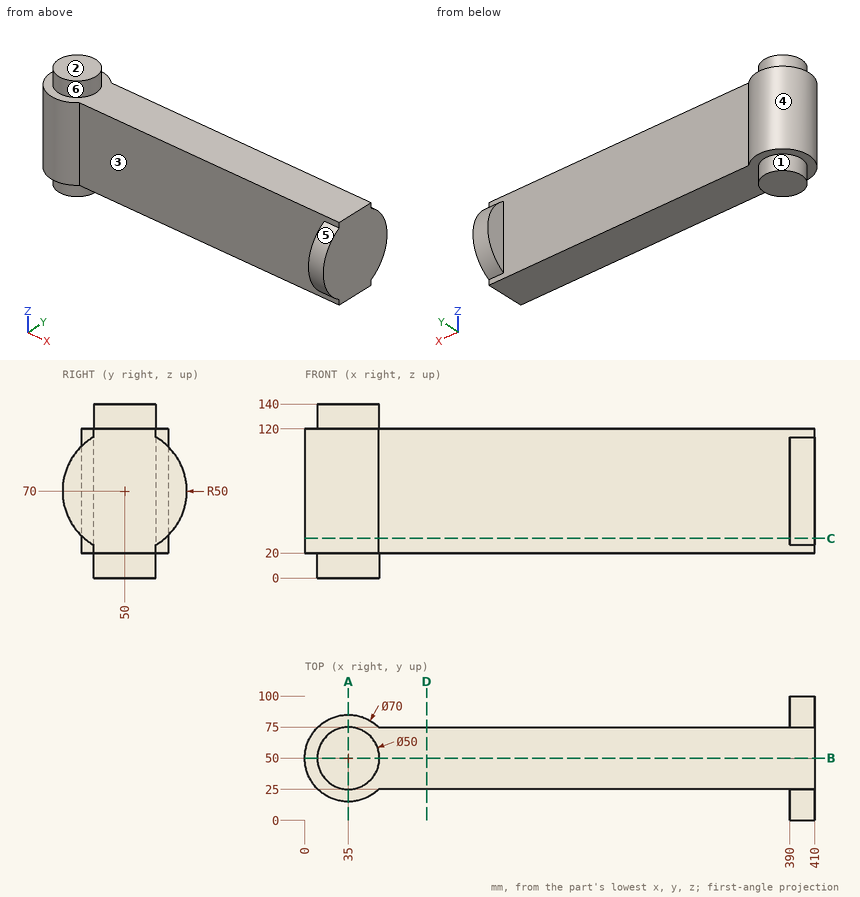
Design review of the part shown in the three views and the two pictorial views. Dimensions are in mm from the part's minimum x, y and z. A direction names the side the tool comes from. Round coordinates to 2 decimals unless told otherwise and drop trailing zeros. Write each loop counter-clockwise with the first axis right and the second up, starting at its lowest first coordinate (ties: lowest second). Pieces come first, ordered by that corner, then holes. Notation, with made-up numbers: (27, 44) -> (77, 44) arc R32 ccw to (77, 70) -> close; hole circle Ø8 at (66, 54). An arc over 180 degrees is marked (long way). Answer as a JSON object with one key per item and string values.
1. We need section C-C on z = 32. State the section outline as (x, y) points.
Results found:
{"outline": "(59.49, 25) -> (390, 25) -> (390, 17.5) -> (410, 17.5) -> (410, 82.5) -> (390, 82.5) -> (390, 75) -> (59.49, 75) arc R35 ccw (long way) to start"}
2. The part is to be moulded in two halves that separate along X. For the marked faces 1, 2 and 3, say which applies: pulls with the +X half, pulls with the -X half, needs draft (parallel to the pull), parting line crosses it, or undercut.
Results found:
{"face 1": "parting line crosses it", "face 2": "needs draft", "face 3": "undercut"}
3. We need section B-B on y = 50. State the section outline as (x, z) points, and give its area (3 significant figures).
Results found:
{"outline": "(0, 20) -> (10, 20) -> (10, 0) -> (60, 0) -> (60, 20) -> (410, 20) -> (410, 120) -> (60, 120) -> (60, 140) -> (10, 140) -> (10, 120) -> (0, 120) -> close", "area": "43,000 mm^2"}
4. To check wall thickness, follow line 1 along Z through (x, y) = (192.5, 61); line 2 along Y through (x, z) = (306.5, 94); line 3 along X through (y, z) = (48.5, 30). State the ranges of each line that lie inside material, in increasing order.
Results found:
{"line 1": "z = 20 to 120", "line 2": "y = 25 to 75", "line 3": "x = 0.03 to 410"}
5. We need section D-D on x = 98. State the section outline as (y, z) points, and give its area (3 significant figures).
Results found:
{"outline": "(25, 20) -> (75, 20) -> (75, 120) -> (25, 120) -> close", "area": "5,000 mm^2"}
6. Clearance check with flat-ended pins moving along their axes: pin 1 (8 mm diameter, centred on y = 76, z = 18.5, fed in from -X); pin 2 (8 mm diameter, centred on y = 37.5, z = 121, fed in from -X); pin 3 (20 mm diameter, centred on y = 15.5, z = 71, fed in from -X) (3 decimals). State where each tip first meets the part, or that it passes through.
Results found:
{"pin 1": "stops at x = 8.02", "pin 2": "stops at x = 1.08", "pin 3": "stops at x = 10.005"}
7. Machinability: for the marked faces 4, 5 and 6, which of the approach directions +Z, -Z, +X, -X, +Y, -Y give a long, thin tool a straight path to every point of the face, cutting with its end or side? Answer none if there is none.
Results found:
{"face 4": "+Z, -Z", "face 5": "+X, -Y", "face 6": "+Z"}
8. We need section A-A on x = 35. State the section outline as (y, z) points.
Results found:
{"outline": "(15, 20) -> (25, 20) -> (25, 0) -> (75, 0) -> (75, 20) -> (85, 20) -> (85, 120) -> (75, 120) -> (75, 140) -> (25, 140) -> (25, 120) -> (15, 120) -> close"}
